Geometry: final body of the model. Coordinates: model frame, mm. Face numbers are marked on the shaded views. A direction names the side the tool comes from. Give positions to 0.01 mm unless a question says otherwise; leave off trailing zeros. Write each loop counter-clockwise with the first axis right and the second up, starting at its lowest first coordinate (ties: lowest second). Pieces come first, ordered by that corner, then holes. Notation, with made-up numbers: (-26, 6) -> (-4, 6) arc R20 cw to (-4, 11) -> close; hole circle Ø5 at (70.25, 26). An arc over 180 degrees is marked (long way). Use CSV: the item, a comma, the result in double quotes. Start each with the question number.
1) Section D-D (x = 7). Output: boundary loops of the cut face in (y, z).
2) Set-up query: the marked faces 5, 6, 7, 8 and 9. Return all of +Z, -Z, +X, -X, +Y, -Y with unobstructed straight access to the full face (end or side cutting, diameter ignored); none if empty.
3) Draft query along Z for the marked faces 1, 2, 3 and 4. Return one class per face: pulls with the +Z half, pulls with the -Z half, needs draft (parallel to the pull), parting line crosses it, or undercut.
4) Contact query for flat-ended pins moving along their axis: P1, Ø2, axis at x = -5.5, z = 1.5, coming from the +Y side; P2, Ø4, axis at y = 9.5, z = 1, coming from the +X side; P3, Ø1.8, axis at x = 0, y = 10.5, coming from the +Z side. Output: stop coordinate, or through.
5) Section A-A (x = 0). Output: boundary loops of the cut face in (y, z).
6) Section B-B (y = 10.12). Output: boundary loops of the cut face in (x, z), plus the area to 3 significant figures.
7) Section C-C (z = 0.25). Output: boundary loops of the cut face in (x, y), plus the area to 3 significant figures.
8) Material intervals for line 1 (Y direction, x = 0, z = 2.7); line 2 (X direction, y = 0.8, z = 0); line 3 (Z direction, x = 6, y = 1.1), sorted ascending. Write a range as [from, to].
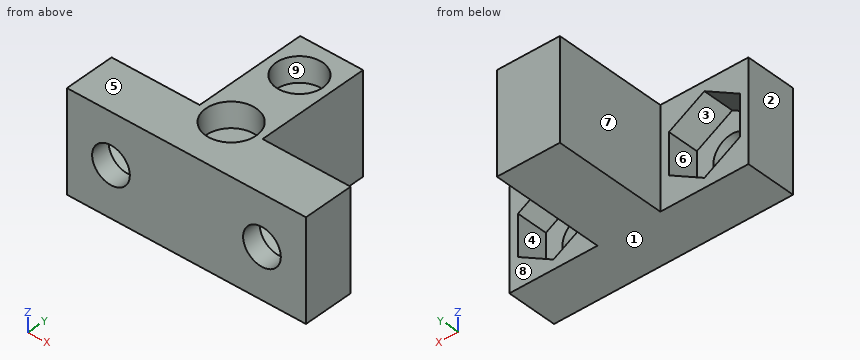
Autodesk Inventor part; units mm, degrees
ref_plane "YZ Plane" through (0, 0, 0) normal (1, 0, 0) x (0, 1, 0)
ref_plane "XZ Plane" through (0, 0, 0) normal (0, 1, 0) x (-1, 0, 0)
ref_plane "XY Plane" through (0, 0, 0) normal (0, 0, 1) x (1, 0, 0)
sketch "Sketch1" plane through (0, 0, 0) normal (0, 1, 0) x (-1, 0, 0)
  line L0 (13.3, 0) -> (-13.3, 0)
  line L1 (0, -6.3) -> (0, 6.3)
  line L2 (-9.5, 4) -> (9.5, 4)
  line L3 (9.5, 4) -> (9.5, -4)
  line L4 (9.5, -4) -> (-9.5, -4)
  line L5 (-9.5, -4) -> (-9.5, 4)
  line L6 (-9.5, 4) -> (9.5, -4) construction
  line L7 (9.5, 4) -> (-9.5, -4) construction
  point P0 (0, 0)
  dimension "d0" = 19
  dimension "d1" = 8
extrude "Extrusion1" add sketch "Sketch1" along normal blind 13
sketch "Sketch2" plane through (-9.5, 0, 4) normal (0, 0, 1) x (1, 0, 0)
  line L0 (19, 0) -> (0, 0)
  line L1 (7, 13) -> (12, 13)
  line L2 (12, 13) -> (12, 0)
  line L3 (12, 0) -> (7, 0)
  line L4 (7, 0) -> (7, 13)
  line L5 (7, 13) -> (12, 0) construction
  line L6 (12, 13) -> (7, 0) construction
  line L7 (0, 13) -> (19, 13)
  line L8 (0, 0) -> (0, 13)
  line L9 (19, 0) -> (19, 13)
  circle A0 centre (9.5, 10.12) radius 1.85
  circle A1 centre (9.5, 4) radius 2
  point P0 (9.5, 0)
  point P1 (9.5, 6.5)
  dimension "d6" = 7
  dimension "d7" = 3.7
  dimension "d8" = 4
  dimension "d9" = 2.5
  dimension "d10" = 2.5
  dimension "d11" = 2
  dimension "d12" = 6.12
  dimension "d19" = 2.5
extrude "Extrusion2" cut sketch "Sketch2" against normal blind 2 contours A0 | A1
sketch "Sketch3" plane through (0, 13, 0) normal (0, 1, 0) x (1, 0, 0)
  line L0 (-9.5, -4) -> (9.5, -4)
  line L1 (2.5, -4) -> (2.5, 4)
  line L2 (9.5, 4) -> (-9.5, 4)
  line L3 (9.5, -4) -> (9.5, 4)
  point P0 (0, 0)
  dimension "d15" = 7
extrude "Extrusion3" cut sketch "Sketch3" against normal blind 9
sketch "Sketch4" plane through (0, 4, 0) normal (0, 1, 0) x (1, 0, 0)
  line L0 (6, -3.25) -> (3.1854, -1.625)
  line L1 (3.1854, -1.625) -> (3.1854, 1.625)
  line L2 (3.1854, 1.625) -> (6, 3.25)
  line L3 (6, 3.25) -> (8.8146, 1.625)
  line L4 (8.8146, 1.625) -> (8.8146, -1.625)
  line L5 (8.8146, -1.625) -> (6, -3.25)
  line L6 (9.5, -4) -> (2.5, -4)
  line L7 (9.5, 4) -> (9.5, -4)
  line L8 (2.5, 4) -> (9.5, 4)
  point P0 (0, 0)
  point P1 (6, 0)
  dimension "d18" = 6.5
  dimension "d23" = 3.5
  dimension "d24" = 4
  dimension "d32" = 5.6292
  dimension "d33" = 6.5
sketch "Sketch7" plane through (0, 13, 0) normal (0, 1, 0) x (1, 0, 0)
  line L0 (-9.5, -4) -> (2.5, -4)
  line L1 (-2.5, -4) -> (-2.5, 4)
  line L2 (2.5, 4) -> (-9.5, 4)
  line L3 (-9.5, 4) -> (-9.5, -4)
  line L4 (-2.5, -4) -> (-9.5, -4)
  line L5 (-9.5, 4) -> (-2.5, 4)
  point P0 (0, 0)
  dimension "d25" = 7
extrude "Extrusion5" cut sketch "Sketch7" against normal blind 9
sketch "Sketch8" plane through (0, 4, 0) normal (0, 1, 0) x (1, 0, 0)
  line L0 (-3.1854, -1.625) -> (-6, -3.25)
  line L1 (-6, -3.25) -> (-8.8146, -1.625)
  line L2 (-8.8146, -1.625) -> (-8.8146, 1.625)
  line L3 (-8.8146, 1.625) -> (-6, 3.25)
  line L4 (-6, 3.25) -> (-3.1854, 1.625)
  line L5 (-3.1854, 1.625) -> (-3.1854, -1.625)
  line L6 (-2.5, 4) -> (-2.5, -4)
  line L7 (-9.5, -4) -> (-9.5, 4)
  line L8 (-9.5, 4) -> (-2.5, 4)
  point P0 (0, 0)
  point P1 (-6, 0)
  dimension "d28" = 6.5
  dimension "d30" = 3.5
  dimension "d31" = 4
  dimension "d34" = 5.6292
sketch "Sketch9" plane through (0, 4, 0) normal (0, 1, 0) x (1, 0, 0)
  circle A0 centre (-6, 0) radius 1.5
  line L0 (-2.5, -4) -> (-9.5, -4)
  line L1 (-2.5, 4) -> (-2.5, -4)
  point P0 (0, 0)
  dimension "d35" = 3
  dimension "d36" = 4
  dimension "d37" = 3.5
extrude "Extrusion6" cut sketch "Sketch4" against normal blind 2.5
sketch "Sketch10" plane through (0, 1.5, 0) normal (0, 1, 0) x (1, 0, 0)
  circle A0 centre (6, 0) radius 1.5
  line L0 (9.5, -4) -> (2.5, -4)
  line L1 (9.5, 4) -> (9.5, -4)
  point P0 (0, 0)
  dimension "d40" = 3
  dimension "d41" = 4
  dimension "d42" = 3.5
extrude "Extrusion7" cut sketch "Sketch10" against normal through all
extrude "Extrusion8" cut sketch "Sketch8" against normal blind 2.5
extrude "Extrusion9" cut sketch "Sketch9" against normal through all
properties part number "uchwyt_drazki_wersja_2"
Answers follow:
1,outline,"(0, -4) -> (4, -4) -> (4, -2.67) -> (1.5, -2.67) -> (1.5, -1.12) -> (0, -1.12) -> close; (0, 1.12) -> (1.5, 1.12) -> (1.5, 2.67) -> (4, 2.67) -> (4, 4) -> (0, 4) -> close"
2,face 5,"+Z, +X, -X, +Y, -Y"
2,face 6,"+Y"
2,face 7,"+Z, -Z, -X, +Y"
2,face 8,"+Z, -Z, +X, +Y"
2,face 9,"+Z"
3,face 1,"pulls with the -Z half"
3,face 2,"needs draft"
3,face 3,"undercut"
3,face 4,"undercut"
4,P1,"stops at y = 1.5"
4,P2,"stops at x = 2.5"
4,P3,"stops at z = 2"
5,outline,"(0, -4) -> (13, -4) -> (13, 4) -> (11.97, 4) -> (11.97, 2) -> (8.27, 2) -> (8.27, 4) -> (6, 4) -> (6, 2) -> (2, 2) -> (2, 4) -> (0, 4) -> close"
6,outline,"(-2.5, -4) -> (2.5, -4) -> (2.5, 4) -> (1.85, 4) -> (1.85, 2) -> (-1.85, 2) -> (-1.85, 4) -> (-2.5, 4) -> close"
6,area,"32.6 mm^2"
7,outline,"(-9.5, 0) -> (-7.48, 0) -> (-7.48, 1.5) -> (-8.81, 1.5) -> (-8.81, 4) -> (-9.5, 4) -> close; (-4.52, 0) -> (4.52, 0) -> (4.52, 1.5) -> (3.19, 1.5) -> (3.19, 4) -> (2.5, 4) -> (2.5, 13) -> (-2.5, 13) -> (-2.5, 4) -> (-3.19, 4) -> (-3.19, 1.5) -> (-4.52, 1.5) -> close; (7.48, 0) -> (9.5, 0) -> (9.5, 4) -> (8.81, 4) -> (8.81, 1.5) -> (7.48, 1.5) -> close"
7,area,"84.0 mm^2"
8,line 1,"y = [0, 2], [6, 8.27], [11.97, 13]"
8,line 2,"x = [-9.5, -7.5], [-4.5, 4.5], [7.5, 9.5]"
8,line 3,"z = [-4, -1.5], [1.5, 4]"
